Design review of the part built by this model. Coordinates are the model's own, in mm. A direction names the side the tool comes from. Coordinates: 2 decimals unless noted, no trailing zeros. Loops run counter-clockwise (first coordinate to the right, second up) from the corner with the lowest first, then second, coordinate; pieces in that order, holes last.
Q1. Add section B-B on z = 8.5. Give the boundary of the cut face in (x, y), and give its area (3 significant figures).
Q2. Wall thickness on probe 1 along Z at (x, y) = (1, 3.75); probe 2 along X at (y, z) = (1.5, 13.5); probe 3 along X at (y, z) = (-0.75, 13): over which ranges is each line inside the solid? List them lowest first.
Q3. Machinability: for faces 5 (the face through (8.25, 3, 0)), 6 (the face through (-7.75, 0, 0)), which of the approach directions +Z, -Z, +X, -X, +Y, -Y give a long, thin tool a straight path to every point of the face, cutting with its end or side? Answer none if there is none.
Q4. Add section A-A on y = 1. Give the boundary of the cut face in (x, z), and give its area (4 significant figures).
Q5. Add section C-C on x = 0.75. Give the boundary of the cut face in (y, z).
Q6. Add section D-D on y = -4. Give the boundary of the cut face in (x, z), and give its area (3 significant figures).
Q7. For P1, Ø1, axis at y = -3.5, z = -13, coming from the +X side; P2, Ø1.5, axis at y = -3, z = -14.5, coming from the +X side; P3, Ø3, axis at y = -1.5, z = 5.5, coming from the +X side, all flat-tipped, find the tip position at first contact; note any pin that passes through.
Q8. Draft analysis for pull direction X (two halves, no side actions). For faces 1 (the face through (0, 0, -20.25)), 2 (the face through (-8, -5, 0)), 3 (the face through (-8.25, 0, 0)), 4 (the face through (7.964, -2.253, 0.291)), state which applies: released by +X, released by -X, zero draft, split by the parting line, or undercut.
```python
from build123d import *

# Parameters (mm, degrees)
F0_W     = 16.5
F0_H     = 41.5
F1_DEPTH = 5
F2_W     = 15
F2_H     = 40.5
F3_DEPTH = 12.5
F5_DEPTH = 22.8


with BuildPart() as f1:
    # F0 (on Front) → F1 (new body, symmetric)
    with BuildSketch(Plane.XZ):
        Rectangle(F0_W, F0_H)
    extrude(amount=F1_DEPTH, both=True)

    # F2 (on Front) → F3 (cut, symmetric)
    with BuildSketch(Plane.XZ):
        with Locations((-0.25, 0)):
            Rectangle(F2_W, F2_H)
    extrude(amount=F3_DEPTH, both=True, mode=Mode.SUBTRACT)

    # F4 (on Top) → F5 (cut, symmetric)
    with BuildSketch(Plane.XY):
        Polygon((10.645687, 0.322955), (8.267023, 0.577699), (7.596283, -5.685302), (10.645687, -6.162507), align=None)
    extrude(amount=F5_DEPTH, both=True, mode=Mode.SUBTRACT)


solid = f1.part
```
Entries:
1. outline: (-8.25, -5) - (-7.75, -5) - (-7.75, 5) - (-8.25, 5) - close; (7.25, -5) - (7.67, -5) - (8.25, 0.42) - (8.25, 5) - (7.25, 5) - close
1. area: 13.4 mm2
2. probe 1: z = -20.75 to -20.25, 20.25 to 20.75
2. probe 2: x = -8.25 to -7.75, 7.25 to 8.25
2. probe 3: x = -8.25 to -7.75, 7.25 to 8.12
3. face 5: +Z, -Z, +X, +Y, -Y
3. face 6: +Y, -Y
4. outline: (-8.25, -20.75) - (8.25, -20.75) - (8.25, 20.75) - (-8.25, 20.75) - close; hole (-7.75, -20.25) - (7.25, -20.25) - (7.25, 20.25) - (-7.75, 20.25) - close
4. area: 77.25 mm2
5. outline: (-5, -20.75) - (5, -20.75) - (5, -20.25) - (-5, -20.25) - close; (-5, 20.25) - (5, 20.25) - (5, 20.75) - (-5, 20.75) - close
6. outline: (-8.25, -20.75) - (7.78, -20.75) - (7.78, 20.75) - (-8.25, 20.75) - close; hole (-7.75, -20.25) - (7.25, -20.25) - (7.25, 20.25) - (-7.75, 20.25) - close
6. area: 57.6 mm2
7. P1: stops at x = 7.88
7. P2: stops at x = 7.96
7. P3: stops at x = 8.21
8. face 1: undercut
8. face 2: zero draft
8. face 3: released by -X
8. face 4: released by +X
